Autodesk Inventor part; units mm, degrees
ref_plane "Arbeitsebene1" through (-5, -7, -5.9) normal (0, 0, 1) x (1, 0, 0)
ref_plane "YZ Plane" through (0, 0, 0) normal (1, 0, 0) x (0, 1, 0)
ref_plane "XZ Plane" through (0, 0, 0) normal (0, 1, 0) x (-1, 0, 0)
sketch "Skizze1" plane through (0, 0, 0) normal (0, 1, 0) x (-1, 0, 0)
  point P0 (0, 0)
sketch "Skizze2" plane through (0, 0, 0) normal (0, 0, 1) x (1, 0, 0)
  circle A0 centre (0, 0) radius 5.85
  dimension "d0" = 11.7
extrude "Extrusion1" add sketch "Skizze2" along normal blind 5 draft -2
sketch "Skizze3" plane through (0, 0, 0) normal (0, 0, -1) x (-1, 0, 0)
  circle A0 centre (0, 0) radius 7.5
  dimension "d3" = 15
extrude "Extrusion2" add sketch "Skizze3" along normal blind 1
sketch "Skizze4" plane through (0, 0, -1) normal (0, 0, -1) x (-1, 0, 0)
  circle A0 centre (0, 0) radius 7.5
ref_plane "Arbeitsebene1" through (-5, -7, -5.9) normal (0, 0, 1) x (1, 0, 0)
extrude "Extrusion3" add sketch "Skizze4" along normal blind 4
chamfer "Fase1" distance 1 angle 45 1 edges at (7.5, 0, 0)
sketch "Skizze5" plane through (0, 0, 0) normal (1, 0, 0) x (0, 1, 0)
  line L0 (-7.5, -1) -> (-7.5, -5)
  line L1 (-7.5, -3) -> (2.9599, -3)
  line L2 (2.9599, -3) -> (7.8543, 1.8945)
  line L3 (7.8543, 1.8945) -> (7.8543, -11.1641)
  line L4 (7.8543, -11.1641) -> (-9.215, -10.2828)
  line L5 (-9.215, -10.2828) -> (-7.5, -3)
  point P0 (0, 0)
  dimension "d11" = 135
extrude "Extrusion4" cut sketch "Skizze5" along normal through all both and the other way through all
properties part number "tmp_20_Cube_Insert_Kinematic_Astromedia_30x40x90_pro_magnetic_M12lens_mirrormount"
For this review, take the finished solid that the model builds, in its own axes (mm). Coordinates: 2 decimals unless noted, no trailing zeros. Loops run counter-clockwise (first coordinate to the right, second up) from the corner with the lowest first, then second, coordinate; pieces in that order, holes last. Notation, with made-up numbers: (-30, 49.25) - (-3, 49.25) arc R17 cw to (-3, 62.25) - close; hole circle Ø8 at (-39.5, 22.5). An arc over 180 degrees is marked (long way). Use one line per item in the form item = value. Start each with the question number.
1) Take a section at C-C (z = 1.75). State the section outline as (x, y) points, plus the area to 3 significant figures.
2) Take a section at B-B (y = 0). State the section outline as (x, z) points.
3) Take a section at D-D (z = 4). State the section outline as (x, y) points, plus the area to 3 significant figures.
4) To check wall thickness, follow probe 1 along Z at (x, y) = (5.5, -3); probe 2 along Y at (x, z) = (3.25, -2.5); probe 3 along X at (y, z) = (1.5, 1). State the ranges of each line that lie inside material, in increasing order. Write a range as from..to.
5) For pin 1 (3 mm diameter, centred on x = -5.5, z = -1, fed in from +Y); pin 2 (4 mm diameter, centred on x = -5.5, y = 3, fed in from +Z); pin 3 (1 mm diameter, centred on x = 1, z = 2.5, fed in from +Y), all flat-tipped, find the tip position at first contact; note any pin that passes through.
6) Take a section at A-A (x = 0). State the section outline as (y, z) points.
7) Draft analysis for pull direction X (two halves, no side actions). For faces 1 (the face through (-0.75, -5.715, 2.465)), 2 (the face through (1, -6, 0)), state which applies: released by +X, released by -X, zero draft, split by the parting line, or undercut.
From the geometry:
q1.outline = circle Ø11.58 at (0, 0)
q1.area = 105 mm2
q2.outline = (-7.5, -3) - (7.5, -3) - (7.5, -1) - (6.5, 0) - (5.85, 0) - (5.68, 5) - (-5.68, 5) - (-5.85, 0) - (-6.5, 0) - (-7.5, -1) - close
q3.outline = circle Ø11.42 at (0, 0)
q3.area = 102 mm2
q4.probe_1 = -3..0
q4.probe_2 = -6.76..3.46
q4.probe_3 = -5.62..5.62
q5.pin_1 = 5.55
q5.pin_2 = 5
q5.pin_3 = 5.74
q6.outline = (-7.5, -3) - (2.96, -3) - (5.96, 0) - (5.85, 0) - (5.68, 5) - (-5.68, 5) - (-5.85, 0) - (-6.5, 0) - (-7.5, -1) - close
q7.face_1 = split by the parting line
q7.face_2 = zero draft
